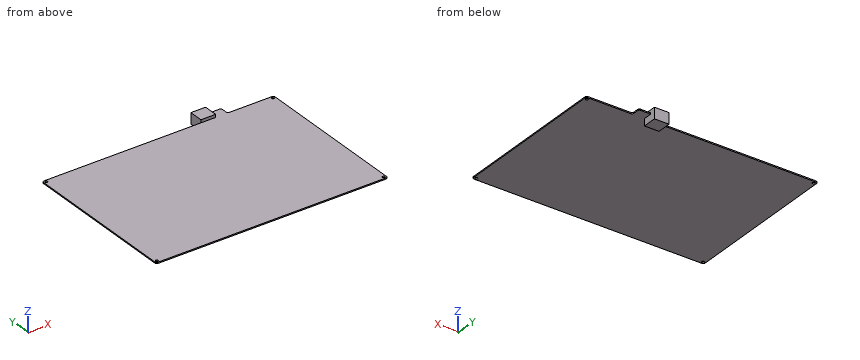
from build123d import *

# Parameters (mm, degrees)
F0_R     = 1.725
F1_DEPTH = 1.6
F3_DEPTH = 19


with BuildPart() as f1:
    # F0 (on Top) → F1 (new body)
    with BuildSketch(Plane.XY):
        with BuildLine():
            ThreePointArc((158, 106), (157.414214, 107.414214), (156, 108))
            Line((156, 108), (96.75, 108))
            ThreePointArc((96.75, 108), (95.335786, 108.585786), (94.75, 110))
            Line((94.75, 110), (94.75, 118))
            ThreePointArc((94.75, 118), (94.164214, 119.414214), (92.75, 120))
            Line((92.75, 120), (58.5, 120))
            Line((58.5, 120), (58.5, 108))
            Line((58.5, 108), (-156, 108))
            ThreePointArc((-156, 108), (-157.414214, 107.414214), (-158, 106))
            Line((-158, 106), (-158, -106))
            ThreePointArc((-158, -106), (-157.414214, -107.414214), (-156, -108))
            Line((-156, -108), (156, -108))
            ThreePointArc((156, -108), (157.414214, -107.414214), (158, -106))
            Line((158, -106), (158, 106))
        make_face()
        with Locations((-154.775, -104.775)):
            Circle(F0_R, mode=Mode.SUBTRACT)
        with Locations((154.775, -104.775)):
            Circle(F0_R, mode=Mode.SUBTRACT)
        with Locations((-154.775, 104.775)):
            Circle(F0_R, mode=Mode.SUBTRACT)
        with Locations((154.775, 104.775)):
            Circle(F0_R, mode=Mode.SUBTRACT)
    extrude(amount=F1_DEPTH)

    # F2 (on face) → F3 (join)
    with BuildSketch(Plane(origin=(0, 108, 0), x_dir=(-1, 0, 0), z_dir=(0, 1, 0))):
        Polygon((-58.5, 1.6), (-58.5, 5.6), (-78.5, 5.6), (-78.5, -9.4), (-58.5, -9.4), (-58.5, 0), align=None)
    extrude(amount=F3_DEPTH)


solid = f1.part
Design review of the part built by this model. Coordinates are the model's own, in mm. Coordinates: 2 decimals unless noted, no trailing zeros. Loops run counter-clockwise (first coordinate to the right, second up) from the corner with the lowest first, then second, coordinate; pieces in that order, holes last. Notation, with made-up numbers: (32, -22.75) - (57, -22.75) arc R38 ccw to (57, 16.25) - close; hole circle Ø1 at (-16, 60). An arc over 180 degrees is marked (long way). Use CSV: the item, a comma, the result in double quotes. Start each with the question number.
1. Clearance check with flat-ended pins moving along their axes: pin 1 (1.8 mm diameter, centred on y = 115.5, z = 1, fed in from +X); pin 2 (5 mm diameter, centred on x = 11, y = -58.5, fed in from -Z); pin 3 (0.8 mm diameter, centred on x = 88.5, z = 1, fed in from +Y). State where each tip first meets the part, or that it passes through.
2. To check wall thickness, follow probe 1 along Z at (x, y) = (45, 0.5); probe 2 along Y at (x, z) = (-88.5, 1.25); probe 3 along Y at (x, z) = (70.5, -7.5). State the ranges of each line that lie inside material, in increasing order.
3. Add section A-A on z = -5.5. Give the boundary of the cut face in (x, y), plus the area to 3 significant figures.
4. Add section B-B on y = 81. Give the boundary of the cut face in (x, z), plus the area to 3 significant figures.
Resolved:
1,pin 1,"x = 94.75"
1,pin 2,"z = 0"
1,pin 3,"y = 120"
2,probe 1,"0 to 1.6"
2,probe 2,"-108 to 108"
2,probe 3,"108 to 127"
3,outline,"(58.5, 108) - (78.5, 108) - (78.5, 127) - (58.5, 127) - close"
3,area,"380 mm2"
4,outline,"(-158, 0) - (158, 0) - (158, 1.6) - (-158, 1.6) - close"
4,area,"506 mm2"
